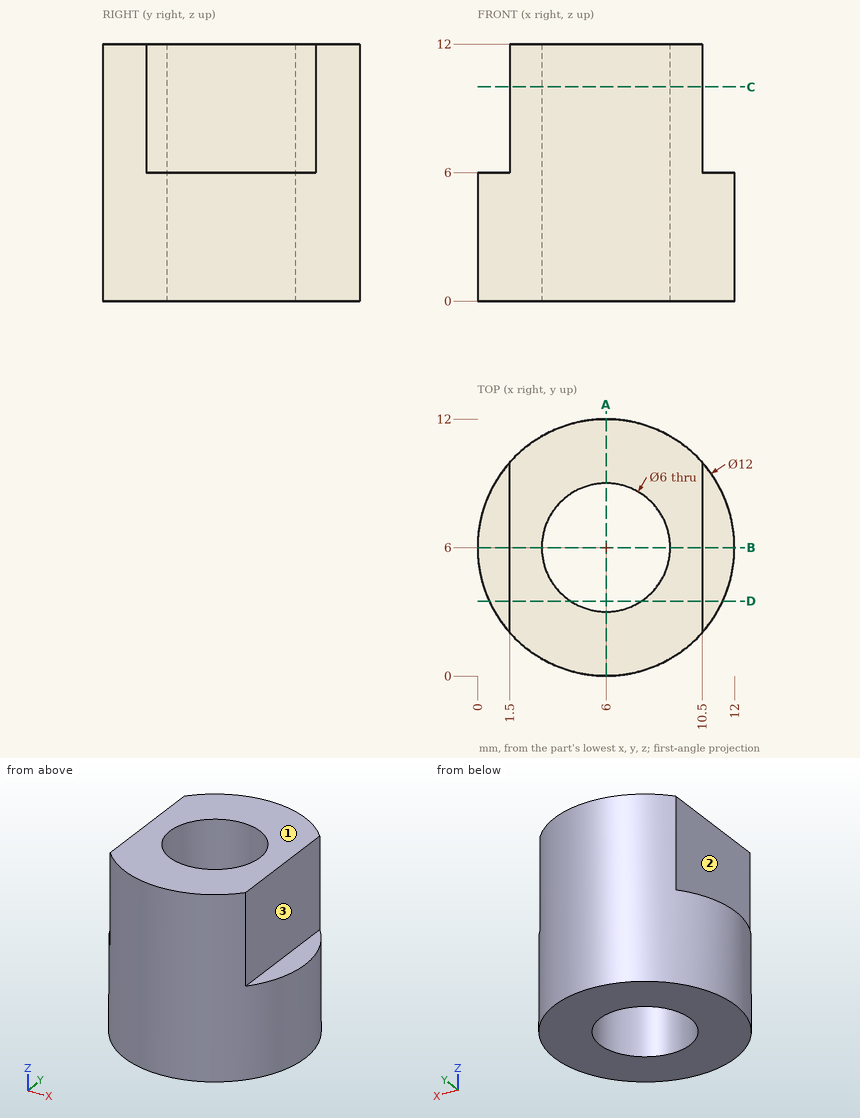
Input: dimensioned drawing with shaded views. Units: mm. Origin: part minimum x, y, z. A direction names the side the tool comes from. Give positions to 0.01 mm unless a question says otherwise; leave off trailing zeros. Order: outer loops, then holes, each group sorted by start corner. A loop starts at its lowest first (then second) coordinate and runs counter-clockwise, first axis right, second up. Notation, with made-up numbers: (-13, 43.25) -> (6, 43.25) arc R22 ccw to (6, 59.25) -> close; hole circle Ø9 at (31.25, -10.75). An arc over 180 degrees is marked (long way). Write item = value, one per line.
Item 1: Contact query for flat-ended pins moving along their axis: pin 1 (3 mm diameter, centred on y = 6, z = 8, fed in from +X); pin 2 (5 mm diameter, centred on y = 5.5, z = 10.5, fed in from -X); pin 3 (6 mm diameter, centred on x = 2.5, z = 9, fed in from -Y). Output: stop coordinate, or through.
Check result:
pin_1 = 10.5
pin_2 = 1.5
pin_3 = 0.02
Item 2: Section query C-C (z = 10). Output: boundary loops of the cut face in (x, y).
Check result:
outline = (1.5, 2.03) arc R6 ccw to (10.5, 2.03) -> (10.5, 9.97) arc R6 ccw to (1.5, 9.97) -> close; hole circle Ø6 at (6, 6)
Item 3: Section query B-B (y = 6). Output: boundary loops of the cut face in (x, z).
Check result:
outline = (0, 0) -> (3, 0) -> (3, 12) -> (1.5, 12) -> (1.5, 6) -> (0, 6) -> close; (9, 0) -> (12, 0) -> (12, 6) -> (10.5, 6) -> (10.5, 12) -> (9, 12) -> close
Item 4: Section query A-A (x = 6). Output: boundary loops of the cut face in (y, z).
Check result:
outline = (0, 0) -> (3, 0) -> (3, 12) -> (0, 12) -> close; (9, 0) -> (12, 0) -> (12, 12) -> (9, 12) -> close
Item 5: Set-up query: the marked faces 1, 2 and 3. Return all of +Z, -Z, +X, -X, +Y, -Y with unobstructed straight access to the full face (end or side cutting, diameter ignored); none if empty.
Check result:
face_1 = +Z, +X, -X, +Y, -Y
face_2 = +Z, -X, +Y, -Y
face_3 = +Z, +X, +Y, -Y
Item 6: Section query D-D (y = 3.5). Output: boundary loops of the cut face in (x, z), then the cut area to 3 significant figures.
Check result:
outline = (0.55, 0) -> (4.34, 0) -> (4.34, 12) -> (1.5, 12) -> (1.5, 6) -> (0.55, 6) -> close; (7.66, 0) -> (11.45, 0) -> (11.45, 6) -> (10.5, 6) -> (10.5, 12) -> (7.66, 12) -> close
area = 79.7 mm²
Item 7: Ray query, probe 1 along Y at (x, z) = (6, 4.5); probe 2 along X at (y, z) = (10.5, 5.25); probe 3 along X at (y, z) = (4.5, 5.5). Return the intervals inside material, ascending.
Check result:
probe_1 = 0 to 3, 9 to 12
probe_2 = 2.03 to 9.97
probe_3 = 0.19 to 3.4, 8.6 to 11.81
